Here's the drawing with two shaded views (mm, measured from the low corner). I have some questions. A direction names the side the tool comes from. Coordinates: 2 decimals unless noted, no trailing zeros. Loops run counter-clockwise (first coordinate to the right, second up) from the corner with the lowest first, then second, coordinate; pieces in that order, holes last. Notation, with made-up numbers: (57.25, 71.25) - (103.25, 71.25) arc R10 ccw to (103.25, 84.25) - close; hole circle Ø3 at (-2.75, -32). An arc over 180 degrees is marked (long way). One line per item, written item: value. Start each with the question number.
(1) On a 3-axis mill with a long thin cutter (end or side, diameter ignored), from which of +Z, -Z, +X, -X, +Y, -Y can I reach the whole of each face in a straight line? I mean the marked faces 4 and 5. Say none if no direction works.
(2) If we section it at C-C on y = 12.25: Write out the boundary of the cut face in (x, z) (3 decimals).
(3) If we mould it in two halves opening along X, with no side actions, what happens to the marked faces 1, 2 and 3? For each: pulls with the +X half, pulls with the -X half, needs draft (parallel to the pull), parting line crosses it, or undercut.
(4) If we section it at D-D on x = 33.5: Write out the boundary of the cut face in (y, z) (3 decimals).
(5) I'm going to push flat-ended pins straight in: P1, Ø6, axis at x = 32.5, y = 15, coming from the +Z side (3 decimals); P2, Ø6, axis at x = 22, z = 15, coming from the +Y side (3 decimals). Where does each tip first touch, or does it pass through?
(6) If we section it at A-A on z = 19.05: Write out the boundary of the cut face in (x, y) (3 decimals), then the cut area to 3 significant figures.
(7) If I drill on line 1 along Y through (x, z) = (12.7, 2.45); line 2 along X through (y, z) = (1.5, 19.05) (3 decimals); line 3 along X through (y, z) = (16.25, 3), over which ranges is the centre line in solid material (lowest first)? Write a range as from..to.
(8) If we section it at B-B on x = 12.5: Write out the boundary of the cut face in (y, z) (1 decimal).
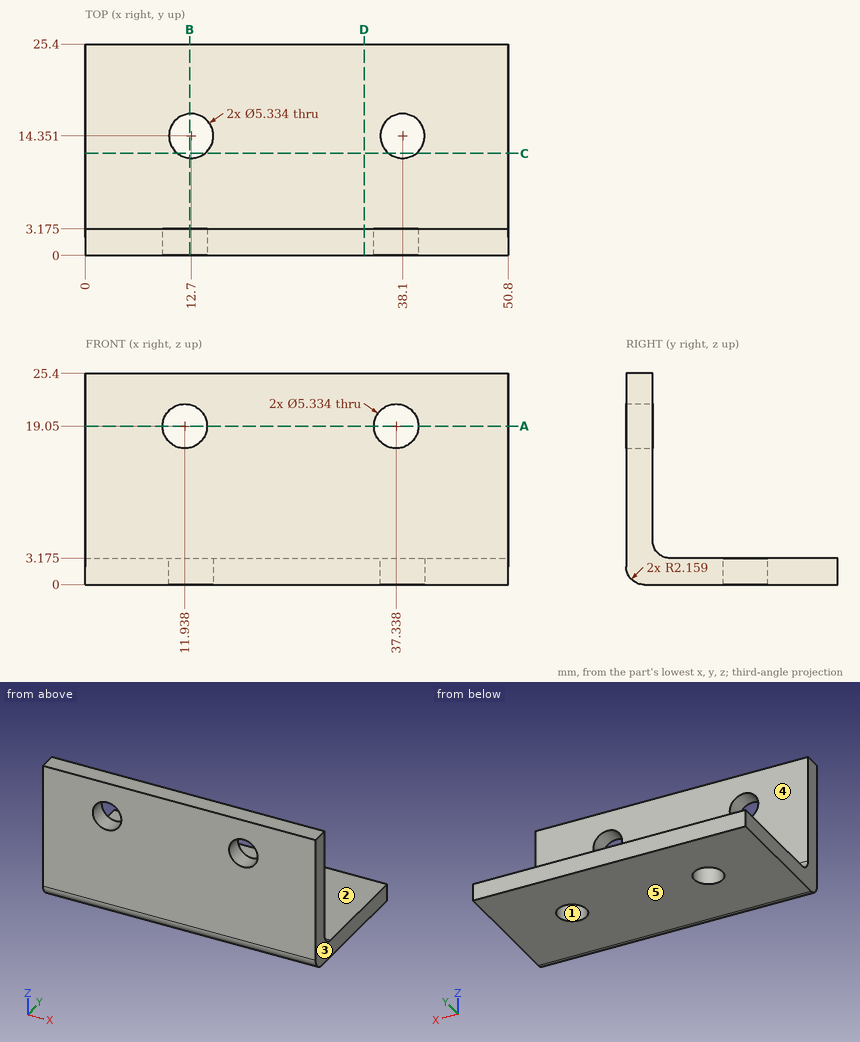
Values:
1. face 4: +Z, +X, -X, +Y
1. face 5: -Z, +X, -X, +Y, -Y
2. outline: (0, 0) - (11.057, 0) - (11.057, 3.175) - (0, 3.175) - close; (14.343, 0) - (36.457, 0) - (36.457, 3.175) - (14.343, 3.175) - close; (39.743, 0) - (50.8, 0) - (50.8, 3.175) - (39.743, 3.175) - close
3. face 1: undercut
3. face 2: needs draft
3. face 3: pulls with the +X half
4. outline: (0, 2.159) arc R2.159 ccw to (2.159, 0) - (25.4, 0) - (25.4, 3.175) - (5.334, 3.175) arc R2.159 cw to (3.175, 5.334) - (3.175, 25.4) - (0, 25.4) - close
5. P1: stops at z = 3.175
5. P2: stops at y = 3.175
6. outline: (0, 0) - (9.271, 0) - (9.271, 3.175) - (0, 3.175) - close; (14.605, 0) - (34.671, 0) - (34.671, 3.175) - (14.605, 3.175) - close; (40.005, 0) - (50.8, 0) - (50.8, 3.175) - (40.005, 3.175) - close
6. area: 127 mm2
7. line 1: y = 0..11.68, 17.02..25.4
7. line 2: x = 0..9.271, 14.605..34.671, 40.005..50.8
7. line 3: x = 0..10.83, 14.57..36.23, 39.97..50.8
8. outline: (0, 2.2) arc R2.2 ccw to (2.2, 0) - (11.7, 0) - (11.7, 3.2) - (5.3, 3.2) arc R2.2 cw to (3.2, 5.3) - (3.2, 16.4) - (0, 16.4) - close; (0, 21.7) - (3.2, 21.7) - (3.2, 25.4) - (0, 25.4) - close; (17, 0) - (25.4, 0) - (25.4, 3.2) - (17, 3.2) - close
